```python
from build123d import *

# Parameters (mm, degrees)
SKETCH_2_W                  = 132
SKETCH_2_H                  = 65
EXTRUDE_2_DEPTH             = 2
SKETCH_2_3_W                = 132
SKETCH_2_3_H                = 65
EXTRUDE_3_DEPTH             = 25
SKETCH_4_R                  = 0.95
SKETCH_4_R_2                = 2
EXTRUDE_4_DEPTH             = 19.5
SKETCH_9_W                  = 6
SKETCH_9_H                  = 2
CUT_EXTRUDE_1_DEPTH         = 23
SKETCH_5_W                  = 8.9
SKETCH_5_H                  = 10
SKETCH_5_W_2                = 6
SKETCH_5_H_2                = 2
CUT_EXTRUDE_2_DEPTH         = 2
SKETCH_11_W                 = 2
SKETCH_11_H                 = 6
CUT_EXTRUDE_3_DEPTH         = 23
SKETCH_12_R                 = 1.6
CUT_EXTRUDE_4_DEPTH         = 23
HOLE_WIZARD_M3_3_D          = 2.5
HOLE_WIZARD_M3_3_DEPTH      = 8.5
HOLE_WIZARD_M3_3_TIP        = 0.751075774
SKETCH_24_W                 = 134
SKETCH_24_H                 = 67
EXTRUDE_5_DEPTH             = 3
SKETCH_25_R                 = 5
EXTRUDE_6_DEPTH             = 31
MACRO_START                 = 30.5
MACRO_FEATURE_1_DEPTH       = 4
MACRO_FEATURE_1_2_DEPTH     = 2
MACRO_START_2               = 45.608387387
MACRO_FEATURE_1_3_OUTLINE_W = 13
MACRO_FEATURE_1_3_OUTLINE_H = 6
MACRO_FEATURE_1_3_DEPTH     = 2.391612613
SKETCH_28_W                 = 4
SKETCH_28_H                 = 10
EXTRUDE_7_DEPTH             = 2
MACRO_START_3               = -10.52248
MACRO_FEATURE_2_DEPTH       = 1.905691985
MACRO_START_4               = -10.216788015
MACRO_FEATURE_2_2_DEPTH     = 1.6
MACRO_START_5               = -13.52599806
MACRO_FEATURE_2_3_DEPTH     = 12.515573406
MACRO_START_6               = -12.373026916
MACRO_FEATURE_2_4_DEPTH     = 10.209631117
MACRO_START_7               = -16
MACRO_FEATURE_2_5_DEPTH     = 10
SKETCH_32_W                 = 59.163412992
SKETCH_32_H                 = 8
EXTRUDE_9_DEPTH             = 2.5
EXTRUDE_10_REACH            = 103.005
SKETCH_31_W                 = 6.738210925
SKETCH_31_H                 = 8.083848138


with BuildPart() as part:
    # 草图2 → 凸台-拉伸2 (new body)
    with BuildSketch(Plane(origin=(0, 0, 0), x_dir=(1, 0, 0), z_dir=(0, 1, 0))):
        Rectangle(SKETCH_2_W, SKETCH_2_H)
    extrude(amount=EXTRUDE_2_DEPTH)

    # 草图2<3> → 凸台-拉伸3 (add)
    with BuildSketch(Plane(origin=(0, 0, 0), x_dir=(1, 0, 0), z_dir=(0, 1, 0))):
        with BuildLine():
            Line((-66, 34.5), (66, 34.5))
            ThreePointArc((66, 34.5), (67.414213562, 33.914213562), (68, 32.5))
            Line((68, 32.5), (68, -32.5))
            ThreePointArc((68, -32.5), (67.414213562, -33.914213562), (66, -34.5))
            Line((66, -34.5), (-66, -34.5))
            ThreePointArc((-66, -34.5), (-67.414213562, -33.914213562), (-68, -32.5))
            Line((-68, -32.5), (-68, 32.5))
            ThreePointArc((-68, 32.5), (-67.414213562, 33.914213562), (-66, 34.5))
        make_face()
        Rectangle(SKETCH_2_3_W, SKETCH_2_3_H, mode=Mode.SUBTRACT)
    extrude(amount=EXTRUDE_3_DEPTH)

    # 草图4 → 凸台-拉伸4 (add)
    with BuildSketch(Plane(origin=(0, 2, 0), x_dir=(1, 0, 0), z_dir=(0, 1, 0))):
        with Locations(Location((63.7, 29.33, 0), (0, 0, 90))):
            Circle(SKETCH_4_R)
        with Locations(Location((63.7, -30.23, 0), (0, 0, 90))):
            Circle(SKETCH_4_R)
        with Locations(Location((-4.6, 29.33, 0), (0, 0, 90))):
            Circle(SKETCH_4_R_2)
        with Locations(Location((-4.6, -30.23, 0), (0, 0, 90))):
            Circle(SKETCH_4_R)
    extrude(amount=EXTRUDE_4_DEPTH)

    # 草图9 → 切除-拉伸1 (cut)
    with BuildSketch(Plane.ZY.offset(68)):
        with Locations((-25.652476361, 14.999984766)):
            Rectangle(SKETCH_9_W, SKETCH_9_H)
        with Locations((-25.652476361, 11.299984766)):
            Rectangle(SKETCH_9_W, SKETCH_9_H)
        with Locations((-25.652476361, 7.599984766)):
            Rectangle(SKETCH_9_W, SKETCH_9_H)
    extrude(amount=-CUT_EXTRUDE_1_DEPTH, mode=Mode.SUBTRACT)

    # 草图5 → 切除-拉伸2 (cut)
    with BuildSketch(Plane(origin=(68, 0, 0), x_dir=(0, 0, -1), z_dir=(1, 0, 0))):
        with Locations((-22.21, 11)):
            Rectangle(SKETCH_5_W, SKETCH_5_H)
        with Locations((25.652457488, 15)):
            Rectangle(SKETCH_5_W_2, SKETCH_5_H_2)
        with Locations((25.652457488, 11.3)):
            Rectangle(SKETCH_5_W_2, SKETCH_5_H_2)
        with Locations((25.652457488, 7.6)):
            Rectangle(SKETCH_5_W_2, SKETCH_5_H_2)
    extrude(amount=-CUT_EXTRUDE_2_DEPTH, mode=Mode.SUBTRACT)

    # 草图11 → 切除-拉伸3 (cut)
    with BuildSketch(Plane.XZ):
        with Locations((-42.109364057, 26.5)):
            Rectangle(SKETCH_11_W, SKETCH_11_H)
        with Locations((-45.609364057, 26.5)):
            Rectangle(SKETCH_11_W, SKETCH_11_H)
        with Locations((-49.109364057, 26.5)):
            Rectangle(SKETCH_11_W, SKETCH_11_H)
        with Locations((-52.609364057, 26.5)):
            Rectangle(SKETCH_11_W, SKETCH_11_H)
        with Locations((-56.109364057, 26.5)):
            Rectangle(SKETCH_11_W, SKETCH_11_H)
        with Locations((-59.609364057, 26.5)):
            Rectangle(SKETCH_11_W, SKETCH_11_H)
    extrude(amount=-CUT_EXTRUDE_3_DEPTH, mode=Mode.SUBTRACT)

    # 草图12 → 切除-拉伸4 (cut)
    with BuildSketch(Plane(origin=(0, 0, -34.5), x_dir=(-1, 0, 0), z_dir=(0, 0, -1))):
        with Locations((-56.73, 20)):
            Circle(SKETCH_12_R)
        with Locations((-44.42, 20)):
            Circle(SKETCH_12_R)
        with Locations((-32.22, 20)):
            Circle(SKETCH_12_R)
    extrude(amount=-CUT_EXTRUDE_4_DEPTH, mode=Mode.SUBTRACT)

    # M3 螺纹孔3
    with Locations(Plane(origin=(0, 21.5, 0), x_dir=(1, 0, 0), z_dir=(0, 1, 0))):
        with Locations((-4.555471055, 29.483622127)):
            Hole(HOLE_WIZARD_M3_3_D / 2, depth=HOLE_WIZARD_M3_3_DEPTH)
            with Locations((0, 0, -(HOLE_WIZARD_M3_3_DEPTH + HOLE_WIZARD_M3_3_TIP / 2))):  # 118° drill point
                Cone(0, HOLE_WIZARD_M3_3_D / 2, HOLE_WIZARD_M3_3_TIP, mode=Mode.SUBTRACT)

    # 草图24 → 凸台-拉伸5 (add)
    with BuildSketch(Plane(origin=(0, 25, 0), x_dir=(1, 0, 0), z_dir=(0, 1, 0))):
        with BuildLine():
            Line((66, -34.5), (-66, -34.5))
            ThreePointArc((-66, -34.5), (-67.414213562, -33.914213562), (-68, -32.5))
            Line((-68, -32.5), (-68, 32.5))
            ThreePointArc((-68, 32.5), (-67.414213562, 33.914213562), (-66, 34.5))
            Line((-66, 34.5), (66, 34.5))
            ThreePointArc((66, 34.5), (67.414213562, 33.914213562), (68, 32.5))
            Line((68, 32.5), (68, -32.5))
            ThreePointArc((68, -32.5), (67.414213562, -33.914213562), (66, -34.5))
        make_face()
        Rectangle(SKETCH_24_W, SKETCH_24_H, mode=Mode.SUBTRACT)
    extrude(amount=EXTRUDE_5_DEPTH)

    # 草图25 → 凸台-拉伸6 (add)
    with BuildSketch(Plane(origin=(0, 2, 0), x_dir=(1, 0, 0), z_dir=(0, 1, 0))):
        with Locations(Location((-40.969280892, 2.451986174, 0), (0, 0, 90))):
            Circle(SKETCH_25_R)
    extrude(amount=EXTRUDE_6_DEPTH)



with BuildPart() as body_2:
    # Macro Feature 1: read off the stored shape, not the designer's step
    # Macro Feature 1 outline → Macro Feature 1 (new body)
    with BuildSketch(Plane.XY.offset(MACRO_START)):
        Polygon((-36.152325447, 32), (-46.152325447, 32), (-46.257141006, 30), (-36.047509888, 30), align=None)
    extrude(amount=MACRO_FEATURE_1_DEPTH)


with BuildPart() as part_1:
    add(part.part)

    add(body_2.part)  # Macro Feature 1 2 merges body 2
    # Macro Feature 1 2 outline → Macro Feature 1 2 (add)
    with BuildSketch(Plane.XY.offset(MACRO_START)):
        Polygon((-36.047509888, 30), (-46.257141006, 30), (-47.724558825, 2), (-34.580092068, 2), align=None)
    extrude(amount=MACRO_FEATURE_1_2_DEPTH)

    # Macro Feature 1 3 outline → Macro Feature 1 3 (cut)
    with BuildSketch(Plane(origin=(0, 0, 0), x_dir=(1, 0, 0), z_dir=(0, 0.707106781186547, 0.707106781186548)).offset(MACRO_START_2)):
        with Locations((-41.5, -2)):
            Rectangle(MACRO_FEATURE_1_3_OUTLINE_W, MACRO_FEATURE_1_3_OUTLINE_H)
    extrude(amount=MACRO_FEATURE_1_3_DEPTH, mode=Mode.SUBTRACT)

    # 草图28 → 凸台-拉伸7 (add)
    with BuildSketch(Plane(origin=(0, 2, 0), x_dir=(1, 0, 0), z_dir=(0, 1, 0))):
        with Locations((-8.9, 7.909574936)):
            Rectangle(SKETCH_28_W, SKETCH_28_H)
    extrude(amount=EXTRUDE_7_DEPTH)

    # Macro Feature 2: read off the stored shape, not the designer's step
    # Macro Feature 2 outline → Macro Feature 2 (add)
    with BuildSketch(Plane.YZ.offset(MACRO_START_3)):
        Polygon((2, -12.909574936), (2, -13.52599806), (24, -12.373026916), (24, -2.163395799), (2, -1.010424654), (2, -2.909574936), (4, -2.909574936), (4, -12.909574936), align=None)
    extrude(amount=MACRO_FEATURE_2_DEPTH)

    # Macro Feature 2 2 outline → Macro Feature 2 2 (add)
    with BuildSketch(Plane.YZ.offset(MACRO_START_4)):
        Polygon((24, -2.163395799), (24, -12.373026916), (26, -12.268211357), (26, -2.268211357), align=None)
    extrude(amount=MACRO_FEATURE_2_2_DEPTH)

    # Macro Feature 2 3 outline → Macro Feature 2 3 (add)
    with BuildSketch(Plane.XY.offset(MACRO_START_5)):
        Polygon((-10.216788015, 24), (-10.216788015, 26), (-15.016788015, 2), (-10.52248, 2), (-10.52248, 24), align=None)
    extrude(amount=MACRO_FEATURE_2_3_DEPTH)

    # Macro Feature 2 4 outline → Macro Feature 2 4 (add)
    with BuildSketch(Plane.XY.offset(MACRO_START_6)):
        Polygon((-8.616788015, 26), (-8.616788015, 24), (-6.616788015, 24), align=None)
    extrude(amount=MACRO_FEATURE_2_4_DEPTH)

    # Macro Feature 2 5 outline → Macro Feature 2 5 (cut)
    with BuildSketch(Plane.YZ.offset(MACRO_START_7)):
        Polygon((2, -13.52599806), (27, -13.52599806), (27, -12.215803578), (26, -12.268211357), align=None)
        Polygon((26, -2.268211357), (27, -2.320619136), (27, -1.010424654), (2, -1.010424654), align=None)
    extrude(amount=MACRO_FEATURE_2_5_DEPTH, mode=Mode.SUBTRACT)

    # 草图32 → 凸台-拉伸9 (add)
    with BuildSketch(Plane.XY.offset(-32.5)):
        with Locations((36.418293504, 10)):
            Rectangle(SKETCH_32_W, SKETCH_32_H)
    extrude(amount=EXTRUDE_9_DEPTH)

    # 草图31 → 凸台-拉伸10 (add, up to next)
    with BuildSketch(Plane(origin=(0, 0, 32.5), x_dir=(-1, 0, 0), z_dir=(0, 0, -1)), mode=Mode.PRIVATE) as extrude_10_sk1:
        with Locations((21.534982766, 6.041924069)):
            Rectangle(SKETCH_31_W, SKETCH_31_H)
    extrude_10_tool1 = extrude(extrude_10_sk1.sketch, amount=EXTRUDE_10_REACH, mode=Mode.PRIVATE) - part_1.part
    add(extrude_10_tool1.solids().sort_by_distance((-21.534983, 6.041924, 32.5))[0])


solid = part_1.part
```
Can you work these out from the model? Positions are in its coordinate system, mm. A direction names the side the tool comes from. Round coordinates to 2 decimals unless told otherwise and drop trailing zeros. Order: outer loops, then holes, each group sorted by start corner. A loop starts at its lowest first (then second) coordinate and runs counter-clockwise, first axis right, second up. Notation, with made-up numbers: (36.5, 81.5) -> (91.5, 81.5) arc R21 cw to (91.5, 89.5) -> close; hole circle Ø8 at (-7, 43.25). An arc over 180 degrees is marked (long way). Return JSON: item names as keys, results as strings. Group by question number.
1. If we section it at B-B, the plane x = 56.73: Write out the boundary of the cut face in (y, z).
2. I need wall thicknesses on line 1 (X direction, y = 4.5, z = 4); line 2 (Z direction, x = -61, y = 3.5); line 3 (Z direction, x = 51, y = 27.5). Which ranges of each line are inside material? Lowest first, please. Write a range as [from, to].
3. Will this pin go through, and if not, where does the flat tip stop? pin 1 (1 mm diameter, centred on x = -67, y = 11, fed in from +Z).
4. If we section it at A-A, the plane z = 22: Write out the boundary of the cut face in (x, y).
5. If we section it at C-C, the plane x = 16: Write out the boundary of the cut face in (y, z), then the cut area to 3 significant figures.
6. If we section it at D-D, the plane z = 13: Write out the boundary of the cut face in (x, y), then the cut area to 3 significant figures.
7. We'd pull the mould along Y, two halves only. Please class faces 1 (the face through (43.56, 21.35, -33.51)), 2 (the face through (-3.383, 11.614, -27.743)), 3 (the face through (-4.58, 12.38, -29.7)): released by +Y, released by -Y, zero draft, split by the parting line, or undercut.
8. Which directions (+Z, -Z, +X, -X, +Y, -Y) give clear straight access to the entire face, cutting with the end or side of a thin tool? Please do faces 4 (the face through (36, 6, -31)), 5 (the face through (-45.185, 17.283, -5.14)), 6 (the face through (-68, 14, 0)).
Output values:
{
 "1": {"outline": "(0, -34.5) -> (18.4, -34.5) -> (18.4, -32.5) -> (14, -32.5) -> (14, -30) -> (6, -30) -> (6, -32.5) -> (2, -32.5) -> (2, 32.5) -> (25, 32.5) -> (25, 33.5) -> (28, 33.5) -> (28, 34.5) -> (0, 34.5) -> close; (21.6, -34.5) -> (28, -34.5) -> (28, -33.5) -> (25, -33.5) -> (25, -32.5) -> (21.6, -32.5) -> close"},
 "2": {"line 1": "[-68, -66], [-24.9, -18.17], [66, 68]", "line 2": "[-34.5, -32.5], [32.5, 34.5]", "line 3": "[-34.5, -33.5], [33.5, 34.5]"},
 "3": {"pin 1": "z = 34.44"},
 "4": {"outline": "(-68, 0) -> (68, 0) -> (68, 6) -> (66, 6) -> (66, 2) -> (-18.17, 2) -> (-18.17, 10.08) -> (-24.9, 10.08) -> (-24.9, 2) -> (-66, 2) -> (-66, 25) -> (-67, 25) -> (-67, 28) -> (-68, 28) -> close; (66, 16) -> (68, 16) -> (68, 28) -> (67, 28) -> (67, 25) -> (66, 25) -> close"},
 "5": {"outline": "(0, -34.5) -> (28, -34.5) -> (28, -33.5) -> (25, -33.5) -> (25, -32.5) -> (14, -32.5) -> (14, -30) -> (6, -30) -> (6, -32.5) -> (2, -32.5) -> (2, 32.5) -> (25, 32.5) -> (25, 33.5) -> (28, 33.5) -> (28, 34.5) -> (0, 34.5) -> close", "area": "256 mm²"},
 "6": {"outline": "(-68, 0) -> (68, 0) -> (68, 28) -> (67, 28) -> (67, 25) -> (66, 25) -> (66, 2) -> (-18.17, 2) -> (-18.17, 10.08) -> (-24.9, 10.08) -> (-24.9, 2) -> (-66, 2) -> (-66, 25) -> (-67, 25) -> (-67, 28) -> (-68, 28) -> close", "area": "424 mm²"},
 "7": {"face 1": "undercut", "face 2": "zero draft", "face 3": "released by +Y"},
 "8": {"face 4": "none", "face 5": "+Y", "face 6": "+Z, -Z, -X, +Y, -Y"}
}
